from build123d import *

# Parameters (mm, degrees)
F1_DEPTH = 10.16


with BuildPart() as f1:
    # F0 (on Top) → F1 (new body)
    with BuildSketch(Plane.XY):
        Polygon((44.45, 0), (31.75, 0), (31.75, -10.16), (10.16, -10.16), (10.16, -19.05), (0, -19.05), (0, -31.75), (10.16, -31.75), (10.16, -44.45), (0, -44.45), (0, -57.15), (10.16, -57.15), (10.16, -69.85), (0, -69.85), (0, -82.55), (10.16, -82.55), (10.16, -95.25), (0, -95.25), (0, -107.95), (10.16, -107.95), (10.16, -120.65), (0, -120.65), (0, -133.35), (10.16, -133.35), (10.16, -146.05), (0, -146.05), (0, -158.75), (10.16, -158.75), (10.16, -167.64), (31.75, -167.64), (31.75, -177.8), (44.45, -177.8), (44.45, -167.64), (57.15, -167.64), (57.15, -177.8), (69.85, -177.8), (69.85, -167.64), (82.55, -167.64), (82.55, -177.8), (95.25, -177.8), (95.25, -167.64), (107.95, -167.64), (107.95, -177.8), (120.65, -177.8), (120.65, -167.64), (133.35, -167.64), (133.35, -177.8), (146.05, -177.8), (146.05, -167.64), (167.64, -167.64), (167.64, -158.75), (177.8, -158.75), (177.8, -146.05), (167.64, -146.05), (167.64, -133.35), (177.8, -133.35), (177.8, -120.65), (167.64, -120.65), (167.64, -107.95), (177.8, -107.95), (177.8, -95.25), (167.64, -95.25), (167.64, -82.55), (177.8, -82.55), (177.8, -69.85), (167.64, -69.85), (167.64, -57.15), (177.8, -57.15), (177.8, -44.45), (167.64, -44.45), (167.64, -31.75), (177.8, -31.75), (177.8, -19.05), (167.64, -19.05), (167.64, -10.16), (146.05, -10.16), (146.05, 0), (133.35, 0), (133.35, -10.16), (120.65, -10.16), (120.65, 0), (107.95, 0), (107.95, -10.16), (95.25, -10.16), (95.25, 0), (82.55, 0), (82.55, -10.16), (69.85, -10.16), (69.85, 0), (57.15, 0), (57.15, -10.16), (44.45, -10.16), align=None)
        with BuildLine():
            ThreePointArc((31.75, -69.85), (33.609872, -65.359872), (38.1, -63.5))
            Line((38.1, -63.5), (139.7, -63.5))
            ThreePointArc((139.7, -63.5), (144.190128, -65.359872), (146.05, -69.85))
            Line((146.05, -69.85), (146.05, -80.645))
            ThreePointArc((146.05, -80.645), (144.190128, -85.135128), (139.7, -86.995))
            Line((139.7, -86.995), (38.1, -86.995))
            ThreePointArc((38.1, -86.995), (33.609872, -85.135128), (31.75, -80.645))
            Line((31.75, -80.645), (31.75, -69.85))
        make_face(mode=Mode.SUBTRACT)
    extrude(amount=F1_DEPTH)


solid = f1.part
The model under review builds one solid part; all positions refer to its coordinate system, in mm. A direction names the side the tool comes from. Give positions to 0.01 mm unless a question says otherwise; leave off trailing zeros. Order: outer loops, then holes, each group sorted by start corner. A loop starts at its lowest first (then second) coordinate and runs counter-clockwise, first axis right, second up. Notation, with made-up numbers: M -10,80 L 37,80 A11 ccw 37,91 Z; hole C -12.5,41 d6. An arc over 180 degrees is marked long. Use one line per item in the form item = value. Start each with the question number.
Item 1: Insertion check: pin 1 Ø5 at (y, z) = (-3, 3.5) entering from +X; pin 2 Ø3 at (x, z) = (6.5, 4) entering from +Y; pin 3 Ø3 at (x, z) = (171, 3.5) entering from -Y. Each pin has a flat end and moves straight along its axis. Give the tip position at first contact, or say it passes through.
Item 2: We need section C-C on y = -110. Give the boundary of the cut face in (x, z).
Item 3: The part is to be moulded in two halves that separate along Y. For faces 1 (the flat face through (114, 0, 5)), 2 (the flat face through (0, -76, 5)), 3 (the flat face through (10.16, -140, 5)), 4 (the flat face through (167.64, -114, 5)), say which applies: pulls with the +Y half, pulls with the -Y half, needs draft (parallel to the pull), parting line crosses it, or undercut.
Item 4: For faces 5 (the flat face through (102, -10.16, 5)), 6 (the cylindrical face through (33.66, -85.184, 5.009)), 7 (the flat face through (157, -10.16, 5)), list the 3-axis set-ups (+Z, -Z, +X, -X, +Y, -Y) from which the entire face can be reached by the end or side of a thin tool; tool diameter is ignored.
Item 5: To check wall thickness, follow line 1 along Y through (x, z) = (134.5, 7) (3 decimals); line 2 along Y through (x, z) = (124, 7.75) (3 decimals); line 3 along Y through (x, z) = (160.5, 1.75). State the ranges of each line that lie inside material, in increasing order. Write a range as from..to.
Item 6: We need section B-B on x = 76. Give the boundary of the cut face in (y, z) (3 decimals).
Item 7: We need section D-D on x = 150. Give the boundary of the cut face in (y, z), plus the area to 3 significant figures.
Item 8: We need section A-A on x = 110.5. Give the boundary of the cut face in (y, z) (3 decimals).
Completed:
q1.pin_1 = 146.05
q1.pin_2 = -19.05
q1.pin_3 = -158.75
q2.outline = M 10.16,0 L 167.64,0 L 167.64,10.16 L 10.16,10.16 Z
q3.face_1 = pulls with the +Y half
q3.face_2 = needs draft
q3.face_3 = undercut
q3.face_4 = undercut
q4.face_5 = +Z, -Z, +Y
q4.face_6 = +Z, -Z
q4.face_7 = +Z, -Z, +X, +Y
q5.line_1 = -177.8..-86.995, -63.5..0
q5.line_2 = -167.64..-86.995, -63.5..-10.16
q5.line_3 = -167.64..-10.16
q6.outline = M -167.64,0 L -86.995,0 L -86.995,10.16 L -167.64,10.16 Z; M -63.5,0 L -10.16,0 L -10.16,10.16 L -63.5,10.16 Z
q7.outline = M -167.64,0 L -10.16,0 L -10.16,10.16 L -167.64,10.16 Z
q7.area = 1,600 mm²
q8.outline = M -177.8,0 L -86.995,0 L -86.995,10.16 L -177.8,10.16 Z; M -63.5,0 L 0,0 L 0,10.16 L -63.5,10.16 Z
